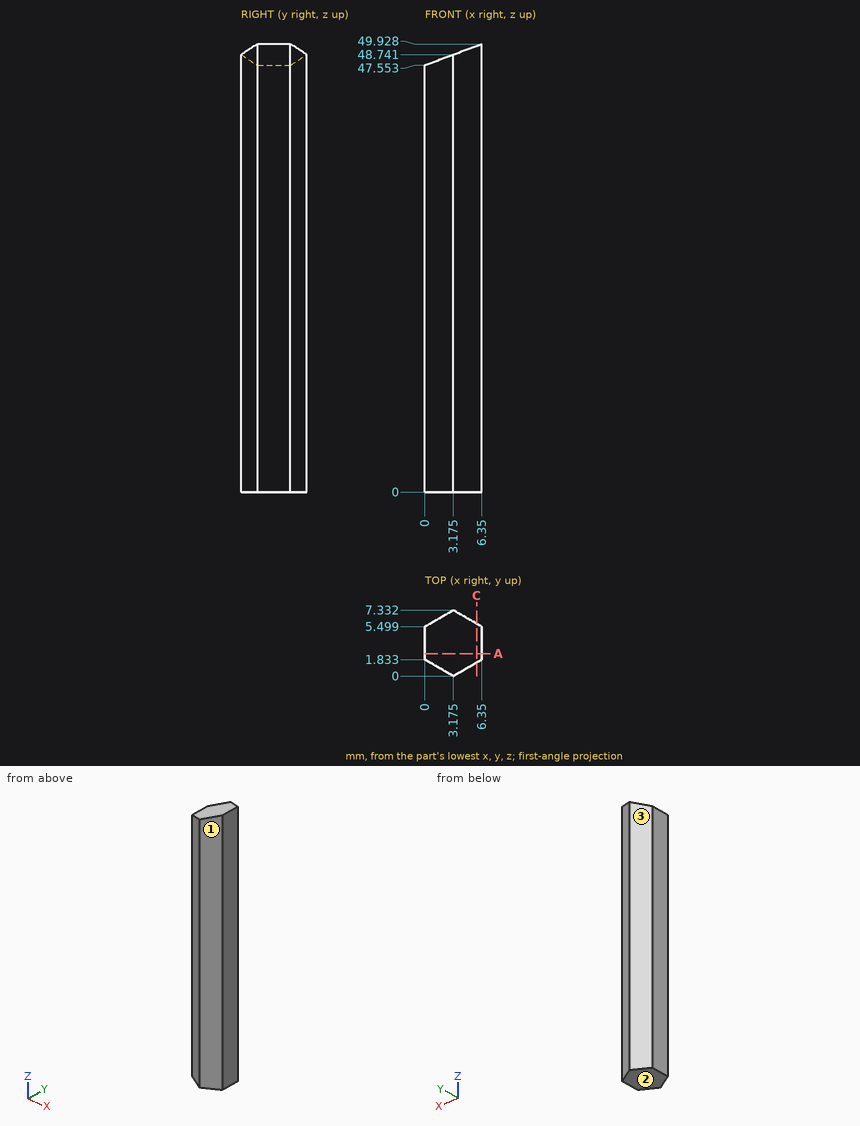
Design review of the part shown in the three views and the two pictorial views. Dimensions are in mm from the part's minimum x, y and z. Round coordinates to 2 decimals unless told otherwise and drop trailing zeros. Write each loop counter-clockwise with the first axis right and the second up, starting at its lowest first coordinate (ties: lowest second). Pieces come first, ordered by that corner, then holes.
1) Take a section at C-C on x = 5.75. Give the boundary of the cut face in (y, z) (1 decimal), then the cut area to 3 significant figures.
Answer below:
outline: (1.5, 0) - (5.8, 0) - (5.8, 49.7) - (1.5, 49.7) - close
area: 217 mm2
2) For line 1 along X through (y, z) = (6, 22.5) (1 decimal); line 2 along Z through (x, y) = (4.5, 1.5) (1 decimal); line 3 along Y through (x, z) = (4.25, 19), list the stretches that pass through material, from the lowest coordinate up.
Answer below:
line 1: x = 0.9 to 5.5
line 2: z = 0 to 49.2
line 3: y = 0.62 to 6.71
3) Take a section at A-A on y = 2.5. Give the boundary of the cut face in (x, z).
Answer below:
outline: (0, 0) - (6.35, 0) - (6.35, 49.93) - (0, 47.55) - close
4) Mouldability with a two-part tool opening along Y and no side actions: class the marked faces 1, 2 and 3 as +Y half, -Y half, draft (parallel to the pull), parting line (faces both ways), or undercut.
Answer below:
face 1: -Y half
face 2: draft
face 3: +Y half
5) Insertion check: pin 1 Ø2 at (x, z) = (1.5, 43.5) entering from -Y. The pin has a flat end and moves straight along its axis. Give the tip position at first contact, or say it passes through.
Answer below:
pin 1: stops at y = 0.39
